```python
from build123d import *

# Parameters (mm, degrees)
SKETCH001_W = 30
SKETCH001_H = 4
PAD_DEPTH   = 4


with BuildPart() as part:
    # Sketch001 → Pad (new body)
    with BuildSketch(Plane.XY):
        with BuildLine():
            Line((0, 90), (0, 128.269605))
            ThreePointArc((51.730395, 180), (15.151482, 164.848518), (0, 128.269605))
            Line((51.730395, 180), (110, 180))
            ThreePointArc((120, 170), (117.071068, 177.071068), (110, 180))
            Line((120, 170), (120, 10))
            ThreePointArc((110, 0), (117.071068, 2.928932), (120, 10))
            Line((110, 0), (51.730395, 0))
            ThreePointArc((0, 51.730395), (15.151482, 15.151482), (51.730395, 0))
            Line((0, 51.730395), (0, 90))
        make_face()
        Polygon((100, 61), (100, 39.5), (83, 39.5), (83, 32.5), (100, 32.5), (100, 11), (110, 11), (110, 61), align=None, mode=Mode.SUBTRACT)
        Polygon((100, 119), (110, 119), (110, 169), (100, 169), (100, 147.5), (83, 147.5), (83, 140.5), (100, 140.5), align=None, mode=Mode.SUBTRACT)
        Polygon((73, 38), (43, 38), (43, 34), (73, 34), (73, 36), align=None, mode=Mode.SUBTRACT)
        Polygon((73, 144), (73, 146), (43, 146), (43, 142), (73, 142), align=None, mode=Mode.SUBTRACT)
        with Locations((58, 158)):
            Rectangle(SKETCH001_W, SKETCH001_H, mode=Mode.SUBTRACT)
        with Locations((58, 22)):
            Rectangle(SKETCH001_W, SKETCH001_H, mode=Mode.SUBTRACT)
    extrude(amount=PAD_DEPTH)


solid = part.part
```
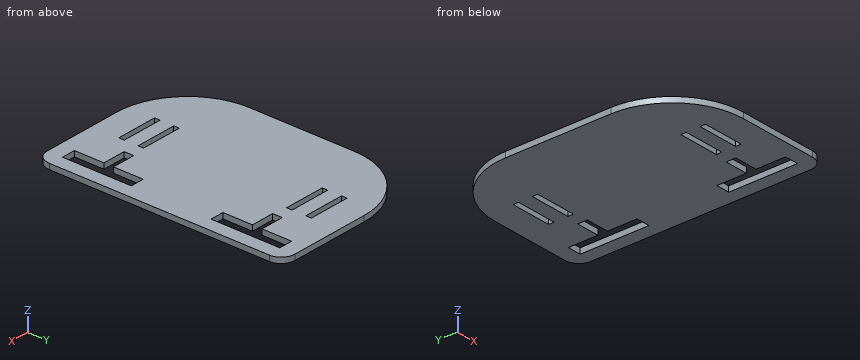
CAD build for the part. Positions are in the model's coordinates, mm. Round coordinates to 2 decimals unless told otherwise and drop trailing zeros. Order: outer loops, then holes, each group sorted by start corner. A loop starts at its lowest first (then second) coordinate and runs counter-clockwise, first axis right, second up. Notation, with made-up numbers: (-22.5, -0.75) - (4.5, -0.75) arc R23 cw to (4.5, 9.25) - close; hole circle Ø11 at (-4, -12.5). An arc over 180 degrees is marked (long way). Answer as CSV lines item,"result". Start each with the question number.
1. Saw through at D-D, the plane y = 137. Write the cut outline in (x, z).
2. Drill centre lines: L1, parallel to Y at x = 89.5, z = 2; L2, parallel to Y at x = 68, z = 1.2; L3, parallel to Y at x = 106, z = 3.7. Where is each one in solid material? Low to high. Write a range as [from, to].
3. Saw through at B-B, the plane y = 15.5. Write the cut outline in (x, z).
4. Saw through at C-C, the plane z = 2.55. Count the separate pieces of the cut face and the enclosed holes in it, and give its area (3 significant figures).
5. Saw through at A-A, the plane x = 55.5. Write the cut outline in (y, z).
6. Pin check, flat tips, straight feed: pin 1 (2 mm diameter, centred on y = 144.5, z = 2, fed in from -X); pin 2 (2 mm diameter, centred on y = 23, z = 1.5, fed in from -X). Stop position of each tip, or through.
Model answer:
1,outline,"(0.74, 0) - (100, 0) - (100, 4) - (0.74, 4) - close; (110, 0) - (120, 0) - (120, 4) - (110, 4) - close"
2,L1,"y = [0, 32.5], [39.5, 140.5], [147.5, 180]"
2,L2,"y = [0, 20], [24, 34], [38, 142], [146, 156], [160, 180]"
2,L3,"y = [0, 11], [61, 119], [169, 180]"
3,outline,"(14.81, 0) - (100, 0) - (100, 4) - (14.81, 4) - close; (110, 0) - (120, 0) - (120, 4) - (110, 4) - close"
4,separate pieces,"1"
4,enclosed holes,"6"
4,area,"18,700 mm²"
5,outline,"(0, 0) - (20, 0) - (20, 4) - (0, 4) - close; (24, 0) - (34, 0) - (34, 4) - (24, 4) - close; (38, 0) - (142, 0) - (142, 4) - (38, 4) - close; (146, 0) - (156, 0) - (156, 4) - (146, 4) - close; (160, 0) - (180, 0) - (180, 4) - (160, 4) - close"
6,pin 1,"stops at x = 2.29"
6,pin 2,"stops at x = 8.06"
